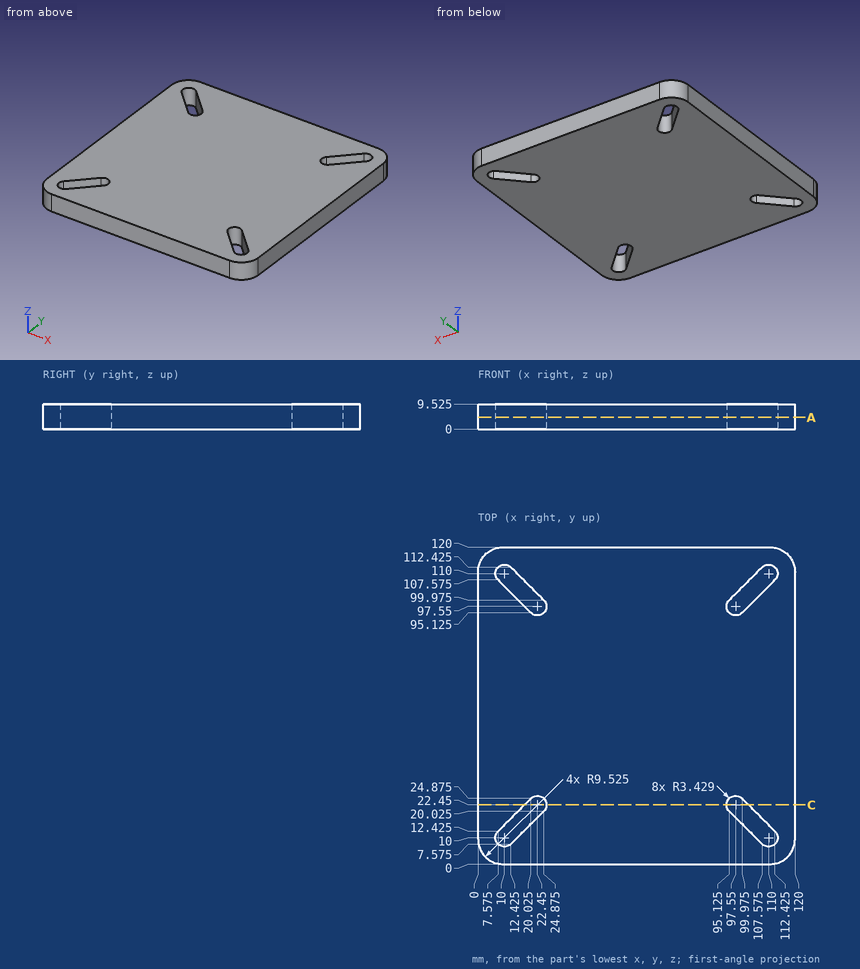
Input: dimensioned drawing with shaded views. Units: mm. Origin: part minimum x, y, z. Round coordinates to 2 decimals unless told otherwise and drop trailing zeros. Loops run counter-clockwise (first coordinate to the right, second up) from the corner with the lowest first, then second, coordinate; pieces in that order, holes last. Notation, with made-up numbers: M 89.25,0.5 L 123.25,0.5 A31 ccw 123.25,27.5 Z; hole C 15.5,-12 d3. An arc over 180 degrees is marked long. Answer in a Markdown table with one row per item. Add a question column.
1. Contact query for flat-ended pins moving along their axis: pin 1 (1 mm diameter, centred on x = 20, y = 16.5, fed in from -Z); pin 2 (4 mm diameter, centred on y = 16, z = 5, fed in from -X). Output: stop coordinate, or through.
2. Section C-C (y = 22.45). Output: boundary loops of the cut face in (x, z) (1 decimal), and give its area (3 significant figures).
3. Ray query, probe 1 along Y at (x, z) = (20, 8.5); probe 2 along X at (y, z) = (7, 6.75); probe 3 along X at (y, z) = (96, 7). Return the intervals inside material, ascending.
4. Section A-A (z = 4.5). Give the number of separate pieces and of enclosed holes in the cut face, and give its area (3 significant figures).
Values follow:
| question | item | result |
|---|---|---|
| 1 | pin 1 | through |
| 1 | pin 2 | x = 0 |
| 2 | outline | M 0,0 L 17.6,0 L 17.6,9.5 L 0,9.5 Z; M 25.9,0 L 94.1,0 L 94.1,9.5 L 25.9,9.5 Z; M 102.4,0 L 120,0 L 120,9.5 L 102.4,9.5 Z |
| 2 | area | 985 mm^2 |
| 3 | probe 1 | 0 to 15.15, 24.85 to 95.15, 104.85 to 120 |
| 3 | probe 2 | 0.34 to 8.34, 11.66 to 108.34, 111.66 to 119.66 |
| 3 | probe 3 | 0 to 19.15, 25.51 to 94.49, 100.85 to 120 |
| 4 | separate pieces | 1 |
| 4 | enclosed holes | 4 |
| 4 | area | 13,700 mm^2 |
